```python
from build123d import *

# Parameters (mm, degrees)
SKETCH_1_W                        = 50
SKETCH_1_H                        = 30
SM_BASE_FLANGE_1_DEPTH            = 3
SM_EDGE_FLANGE_1_STRIP_W          = 13.4732
SM_EDGE_FLANGE_1_STRIP_H          = 3
SM_EDGE_FLANGE_1_STRIP_CUT_DEPTH  = 34
SM_EDGE_FLANGE_1_RELIEF_W         = 14.9732
SM_EDGE_FLANGE_1_RELIEF_H         = 1.5
SM_EDGE_FLANGE_1_RELIEF_CUT_DEPTH = 3
SM_EDGE_FLANGE_1_DEPTH            = 34
CHAMFER_1_SIZE                    = 5
CUT_EXTRUDE_1_DEPTH               = 10


# Sheet-metal steps are written as plain solids
with BuildPart() as part:
    # Sketch 1 → 基体-法兰1 (new body)
    with BuildSketch(Plane.XY):
        with Locations((25, 15)):
            Rectangle(SKETCH_1_W, SKETCH_1_H)
    extrude(amount=-SM_BASE_FLANGE_1_DEPTH)

    # 边线-法兰1 strip (across the edge) → 边线-法兰1 strip cut (cut)
    with BuildSketch(Plane.YZ.offset(8)):
        with Locations((-3, -1.5)):
            Rectangle(SM_EDGE_FLANGE_1_STRIP_W, SM_EDGE_FLANGE_1_STRIP_H)
    extrude(amount=SM_EDGE_FLANGE_1_STRIP_CUT_DEPTH, mode=Mode.SUBTRACT)

    # 边线-法兰1 relief (on the sheet) → 边线-法兰1 relief cut (cut)
    with BuildSketch(Plane(origin=(8, 3.7366, 0), x_dir=(0, 1, 0), z_dir=(0, 0, 1))):
        with Locations((-5.9866, 0.75)):
            Rectangle(SM_EDGE_FLANGE_1_RELIEF_W, SM_EDGE_FLANGE_1_RELIEF_H)
        with Locations((-5.9866, -34.75)):
            Rectangle(SM_EDGE_FLANGE_1_RELIEF_W, SM_EDGE_FLANGE_1_RELIEF_H)
    extrude(amount=-SM_EDGE_FLANGE_1_RELIEF_CUT_DEPTH, mode=Mode.SUBTRACT)

    # 边线-法兰1 section (across the edge) → 边线-法兰1 (add)
    with BuildSketch(Plane.YZ.offset(8)):
        with BuildLine():
            Line((0, 0.7366), (0, 77))
            Line((0, 77), (3, 77))
            Line((3, 77), (3, 0.7366))
            ThreePointArc((3, 0.7366), (3.215745145, 0.215745145), (3.7366, 0))
            Line((3.7366, 0), (3.7366, -3))
            ThreePointArc((3.7366, -3), (1.094424801, -1.905575199), (0, 0.7366))
        make_face()
    extrude(amount=SM_EDGE_FLANGE_1_DEPTH)

    # 倒角1
    chamfer_1_edges = [part.edges().sort_by_distance(p)[0] for p in [
        (8, 1.5, 77),
        (42, 1.5, 77),
        (0, 30, -1.5),
        (50, 30, -1.5),
        (50, 0, -1.5),
        (0, 0, -1.5),
    ]]
    chamfer(chamfer_1_edges, length=CHAMFER_1_SIZE)

    # 草图9 → 切除-拉伸1 (cut)
    with BuildSketch(Plane(origin=(0, 3, 0), x_dir=(1, 0, 0), z_dir=(0, 1, 0))):
        with BuildLine():
            Line((28.5, -29), (28.5, -37))
            ThreePointArc((28.5, -37), (25, -40.5), (21.5, -37))
            Line((21.5, -37), (21.5, -29))
            ThreePointArc((21.5, -29), (25, -25.5), (28.5, -29))
        make_face()
        with BuildLine():
            Line((21.5, -69), (21.5, -61))
            ThreePointArc((21.5, -61), (25, -57.5), (28.5, -61))
            Line((28.5, -61), (28.5, -69))
            ThreePointArc((28.5, -69), (25, -72.5), (21.5, -69))
        make_face()
    extrude(amount=-CUT_EXTRUDE_1_DEPTH, mode=Mode.SUBTRACT)


solid = part.part
```
Source: CAD feature listing. Evaluate the final solid. Frame: model axes, mm. A direction names the side the tool comes from. Round coordinates to 2 decimals unless told otherwise and drop trailing zeros. Write each loop counter-clockwise with the first axis right and the second up, starting at its lowest first coordinate (ties: lowest second). Pieces come first, ordered by that corner, then holes. Notation, with made-up numbers: M 38.5,0 L 66.5,0 A20 cw 66.5,9 Z; hole C 5,24.5 d5. An arc over 180 degrees is marked long. Use CSV: the item, a comma, the result in double quotes. Start each with the question number.
Q1. Line query: line 1 (Z direction, x = 26.5, y = 1.5); line 2 (Y direction, x = 12.5, z = 63); line 3 (Z direction, x = 29, y = 16). Output: solid intervals per line, ascending. Write a range as from..to.
Q2. Cut plane A-A on x = 25. Output: boundary loops of the cut face in (y, z), plus the area to 3 significant figures.
Q3. First-contact query: P1, Ø3.5, axis at y = 2, z = 34.5, coming from the -X side; P2, Ø1.6, axis at x = 7, z = -2, coming from the -Y side; P3, Ø3.5, axis at y = 1.5, z = -1.5, coming from the -X side; P4, Ø9, axis at x = 21, y = 21, coming from the +Z side. Flat tips, straight axial feed; report the tip coordinate or a pass-through.
Q4. Pull-direction query (Z, two-part tool) for faces 1 (the face through (25, 15, -3)), 2 (the face through (40, 1, 74)), 3 (the face through (6.5, 3, -1)), 4 (the face through (24.9, 1.5, 25.5)); classes: +Z half, -Z half, draft (parallel to the pull), parting line (faces both ways), or undercut.
Q5. Cut plane C-C on z = 18.5. Output: boundary loops of the cut face in (x, y).
Q6. Cut plane B-B on x = 38. Output: boundary loops of the cut face in (y, z), plus the area to 3 significant figures.
Q7. Cut plane D-D on y = 27. Output: boundary loops of the cut face in (x, z).
Q8. Access query for faces 5 (the face through (24.76, 1.12, -1.93)), 6 (the face through (21.5, 2, 33)), 7 (the face through (43, 5.237, -1)), 8 (the face through (25, 1, 77)), 9 (the face through (6, 0, -1)). Directions: +Z, -Z, +X, -X, +Y, -Y. A direction counts if a zero-diameter tool reaches every point of the face in a straight line with its end or side. Return the directions, or none.
Results found:
1,line 1,"-2.26..25.84, 40.16..57.84, 72.16..77"
1,line 2,"0..3"
1,line 3,"-3..0"
2,outline,"M 0,0.74 A3.74 ccw 3.74,-3 L 30,-3 L 30,0 L 3.74,0 A0.74 cw 3,0.74 L 3,25.5 L 0,25.5 Z; M 0,40.5 L 3,40.5 L 3,57.5 L 0,57.5 Z; M 0,72.5 L 3,72.5 L 3,77 L 0,77 Z"
2,area,"228 mm^2"
3,P1,"x = 8"
3,P2,"y = 0"
3,P3,"x = 1.75"
3,P4,"z = 0"
4,face 1,"-Z half"
4,face 2,"+Z half"
4,face 3,"draft"
4,face 4,"undercut"
5,outline,"M 8,0 L 42,0 L 42,3 L 8,3 Z"
6,outline,"M 0,0.74 A3.74 ccw 3.74,-3 L 30,-3 L 30,0 L 3.74,0 A0.74 cw 3,0.74 L 3,76 L 0,76 Z"
6,area,"315 mm^2"
7,outline,"M 2,-3 L 48,-3 L 48,0 L 2,0 Z"
8,face 5,"-Z, -Y"
8,face 6,"+Y, -Y"
8,face 7,"+Z, -Z, -Y"
8,face 8,"+Z, +X, -X, +Y, -Y"
8,face 9,"+Z, -Z, +X, -X, -Y"
